The figure shows three views and two pictorial views of one solid part (mm, origin at its lowest corner). Answer the questions. A direction names the side the tool comes from. Round coordinates to 2 decimals unless told otherwise and drop trailing zeros. Write each loop counter-clockwise with the first axis right and the second up, starting at its lowest first coordinate (ties: lowest second). Pieces come first, ordered by that corner, then holes. Notation, with made-up numbers: M 77.5,81 L 114.5,81 A30 cw 114.5,117 Z; hole C 54.25,76.25 d6. An arc over 180 degrees is marked long. Answer in a Markdown table with one row per item.
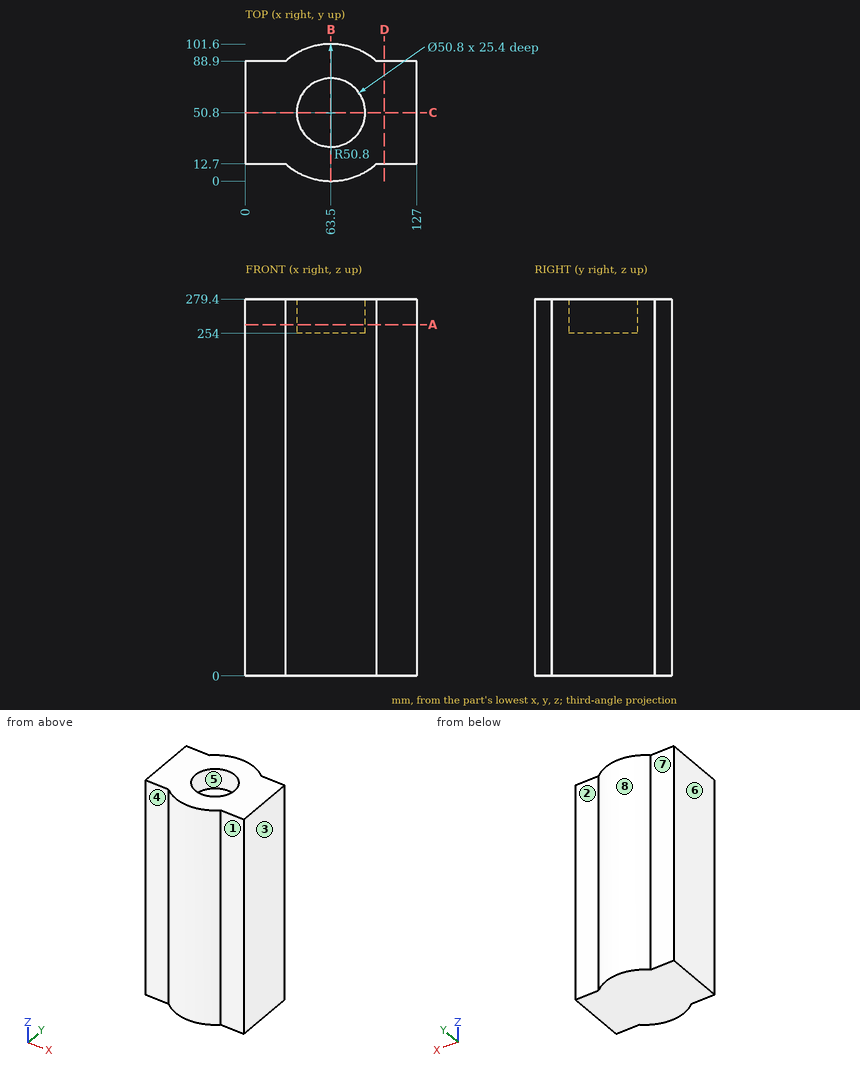
1. Given pin 1 (12 mm diameter, centred on x = 66, z = 61, fed in from -Y); pin 2 (9 mm diameter, centred on x = 109.5, z = 113.5, fed in from -Y); pin 3 (24 mm diameter, centred on x = 18, z = 208, fed in from +Y), each flat-ended and moving along its own axis, determine where each tip first touches the part or whether it passes through.
Calculated:
| item | result |
|---|---|
| pin 1 | stops at y = 0 |
| pin 2 | stops at y = 12.7 |
| pin 3 | stops at y = 88.99 |
2. The part is cut by section D-D (x = 103). Determine the outline of the cut face in (y, z), plus the area to 3 significant figures.
Calculated:
| item | result |
|---|---|
| outline | M 12.7,0 L 88.9,0 L 88.9,279.4 L 12.7,279.4 Z |
| area | 21,300 mm² |
3. The part is cut by section C-C (y = 50.8). Determine the outline of the cut face in (x, z), plus the area to 3 significant figures.
Calculated:
| item | result |
|---|---|
| outline | M 0,0 L 127,0 L 127,279.4 L 88.9,279.4 L 88.9,254 L 38.1,254 L 38.1,279.4 L 0,279.4 Z |
| area | 34,200 mm² |
4. Determine the mould class of the marked faces 5, 6, 7 and 8 for opening direction X: released by +X, released by -X, zero draft, split by the parting line, or undercut.
Calculated:
| item | result |
|---|---|
| face 5 | undercut |
| face 6 | released by -X |
| face 7 | zero draft |
| face 8 | split by the parting line |
5. The part is cut by section A-A (z = 260.5). Determine the outline of the cut face in (x, y), plus the area to 3 significant figures.
Calculated:
| item | result |
|---|---|
| outline | M 0,12.7 L 29.9,12.7 A50.8 ccw 97.1,12.7 L 127,12.7 L 127,88.9 L 97.1,88.9 A50.8 ccw 29.9,88.9 L 0,88.9 Z; hole C 63.5,50.8 d50.8 |
| area | 8,820 mm² |
6. A tool of negligible diameter and unlimited length cuts with its end or side. For the marked faces 1, 2, 3 and 4, from which of +Z, -Z, +X, -X, +Y, -Y can it reach the whole face along a straight path? Write none if from no direction.
Calculated:
| item | result |
|---|---|
| face 1 | +Z, -Z, +X, -Y |
| face 2 | +Z, -Z, +X, +Y |
| face 3 | +Z, -Z, +X, +Y, -Y |
| face 4 | +Z, -Z, -X, -Y |
7. The part is cut by section B-B (x = 63.5). Determine the outline of the cut face in (y, z).
Calculated:
| item | result |
|---|---|
| outline | M 0,0 L 101.6,0 L 101.6,279.4 L 76.2,279.4 L 76.2,254 L 25.4,254 L 25.4,279.4 L 0,279.4 Z |
8. Consider line 1 along Y through (x, z) = (63, 266); line 2 along Y through (x, z) = (116, 183); line 3 along X through (y, z) = (50, 267). Determine where each line is inside the solid, lowest interval first. Write a range as from..to.
Calculated:
| item | result |
|---|---|
| line 1 | y = 0..25.4, 76.2..101.6 |
| line 2 | y = 12.7..88.9 |
| line 3 | x = 0..38.11, 88.89..127 |
